Read the model definition and answer for the solid it produces. Units are mm, in the model's axes. Coordinates: 2 decimals unless noted, no trailing zeros. Write each loop counter-clockwise with the first axis right and the second up, starting at its lowest first coordinate (ties: lowest second). Pieces come first, ordered by that corner, then holes.
Item 1: Section A-A (x = 177) is taken. Give the vertices of the cut face in (y, z).
Item 2: Straight lines are drawn through the part: probe 1 along X at (y, z) = (35, 52.5); probe 2 along Y at (x, z) = (214.5, 45); probe 3 along Z at (x, y) = (-800.1, 36.1). For each, find the intervals that lie inside material, in ascending order.
Item 3: Each of these flat-tipped pins is pushed along its axis until it touches: P1, Ø4.5, axis at x = 520.7, z = 52.98, coming from the -Y side; P2, Ø6, axis at x = -85.5, y = -12, coming from the +Z side. Where does it stop, or does it pass through?
Item 4: Section B-B (y = 6) is taken. Give the vertices of the cut face in (x, z).
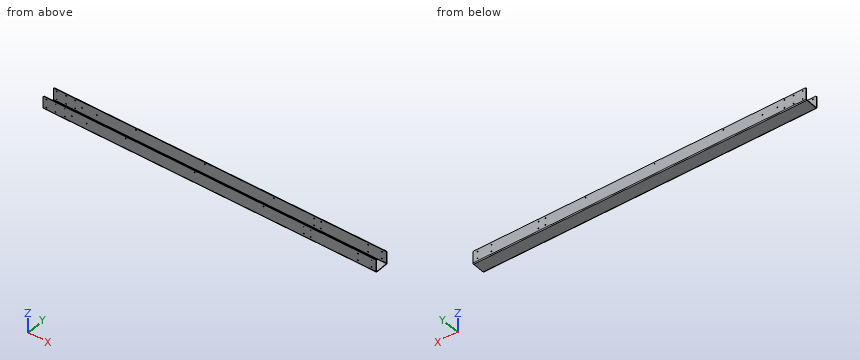
from build123d import *

# Parameters (mm, degrees)
SKETCH2_W                      = 1841.5
SKETCH2_H                      = 69.6722
BASE_FLANGE1_DEPTH             = 3.2639
EDGE_FLANGE1_STRIP_W           = 15.5956
EDGE_FLANGE1_STRIP_H           = 3.2639
EDGE_FLANGE1_STRIP_CUT_DEPTH   = 1841.5
EDGE_FLANGE1_STRIP_2_W         = 15.5956
EDGE_FLANGE1_STRIP_2_H         = 3.2639
EDGE_FLANGE1_STRIP_CUT_2_DEPTH = 1841.5
EDGE_FLANGE1_DEPTH             = 1841.5
EDGE_FLANGE1_BEND_DEPTH        = 1841.5
F_10_0_1935_DIAMETER_HOLE1_D   = 4.9149
F_10_0_1935_DIAMETER_HOLE3_D   = 4.9149
F_10_0_1935_DIAMETER_HOLE4_D   = 4.9149
F_10_0_2_DIAMETER_HOLE1_D      = 5.08
F_10_0_1935_DIAMETER_HOLE6_D   = 4.9149
LPATTERN2_COUNT                = 3
LPATTERN2_PITCH                = 381
FILLET2_R                      = 6.35


# Sheet-metal steps are written as plain solids
with BuildPart() as part:
    # Sketch2 → Base-Flange1 (new body)
    with BuildSketch(Plane.XY):
        Rectangle(SKETCH2_W, SKETCH2_H)
    extrude(amount=-BASE_FLANGE1_DEPTH)

    # Edge-Flange1 strip (across the edge) → Edge-Flange1 strip cut (cut)
    with BuildSketch(Plane(origin=(920.75, 34.8361, 0), x_dir=(0, -1, 0), z_dir=(-1, 0, 0))):
        with Locations((-6.5278, -1.63195)):
            Rectangle(EDGE_FLANGE1_STRIP_W, EDGE_FLANGE1_STRIP_H)
    extrude(amount=EDGE_FLANGE1_STRIP_CUT_DEPTH, mode=Mode.SUBTRACT)

    # Edge-Flange1 strip 2 (across the edge) → Edge-Flange1 strip cut 2 (cut)
    with BuildSketch(Plane(origin=(-920.75, -34.8361, 0), x_dir=(0, 1, 0), z_dir=(1, 0, 0))):
        with Locations((-6.5278, -1.63195)):
            Rectangle(EDGE_FLANGE1_STRIP_2_W, EDGE_FLANGE1_STRIP_2_H)
    extrude(amount=EDGE_FLANGE1_STRIP_CUT_2_DEPTH, mode=Mode.SUBTRACT)

    # Edge-Flange1 section (across the edge) → Edge-Flange1 (add)
    with BuildSketch(Plane(origin=(920.75, 34.8361, 0), x_dir=(0, -1, 0), z_dir=(-1, 0, 0))):
        with BuildLine():
            Line((-3.2639, 1.27), (-3.2639, 66.5861))
            Line((-3.2639, 66.5861), (0, 66.5861))
            Line((0, 66.5861), (0, 1.27))
            ThreePointArc((0, 1.27), (0.371974388, 0.371974388), (1.27, 0))
            Line((1.27, 0), (1.27, -3.2639))
            ThreePointArc((1.27, -3.2639), (-1.935951435, -1.935951435), (-3.2639, 1.27))
        make_face()
    extrude(amount=EDGE_FLANGE1_DEPTH)

    # Edge-Flange1 section 2 (across the edge) → Edge-Flange1 bend (add)
    with BuildSketch(Plane(origin=(-920.75, -34.8361, 0), x_dir=(0, 1, 0), z_dir=(1, 0, 0))):
        with BuildLine():
            Line((-3.2639, 1.27), (-3.2639, 66.5861))
            Line((-3.2639, 66.5861), (0, 66.5861))
            Line((0, 66.5861), (0, 1.27))
            ThreePointArc((0, 1.27), (0.371974388, 0.371974388), (1.27, 0))
            Line((1.27, 0), (1.27, -3.2639))
            ThreePointArc((1.27, -3.2639), (-1.935951435, -1.935951435), (-3.2639, 1.27))
        make_face()
    extrude(amount=EDGE_FLANGE1_BEND_DEPTH)

    # #10 (0.1935) Diameter Hole1 (through all)
    with Locations(Plane(origin=(0, 38.1, 34.8361), x_dir=(-1, 0, 0), z_dir=(0, 1, 0))):
        with Locations((800.1, -23.13305), (800.1, 21.31695), (850.9, 21.31695), (850.9, -23.13305), (901.7, 21.31695), (901.7, -23.13305)):
            Hole(F_10_0_1935_DIAMETER_HOLE1_D / 2)

    # #10 (0.1935) Diameter Hole3 (through all)
    with Locations(Plane(origin=(0, 38.1, 0), x_dir=(1, 0, 0), z_dir=(0, 1, 0))):
        with Locations((819.15, -14.87805), (819.15, -52.97805), (895.35, -14.87805), (895.35, -52.97805)):
            Hole(F_10_0_1935_DIAMETER_HOLE3_D / 2)

    # #10 (0.1935) Diameter Hole4 (through all)
    with Locations(Plane(origin=(0, 38.1, 0), x_dir=(1, 0, 0), z_dir=(0, 1, 0))):
        with Locations((520.7, -14.87805), (558.8, -14.87805), (558.8, -52.97805), (520.7, -52.97805)):
            Hole(F_10_0_1935_DIAMETER_HOLE4_D / 2)

    # #10 (0.2) Diameter Hole1 (through all)
    with Locations(Plane(origin=(0, 38.1, 0), x_dir=(1, 0, 0), z_dir=(0, 1, 0))):
        with Locations((-761.32055, -33.92805), (-678.77055, -33.92805)):
            Hole(F_10_0_2_DIAMETER_HOLE1_D / 2)

    # #10 (0.1935) Diameter Hole6 (through all)
    with Locations(Plane(origin=(0, -38.1, 0), x_dir=(-1, 0, 0), z_dir=(0, -1, 0))):
        with Locations((463.55, -57.0611)):
            f_10_0_1935_diameter_hole6 = Hole(F_10_0_1935_DIAMETER_HOLE6_D / 2)

    # LPattern2: #10 (0.1935) Diameter Hole6 ×3
    with Locations(*[(i * LPATTERN2_PITCH, 0, 0) for i in range(1, LPATTERN2_COUNT)]):
        add(f_10_0_1935_diameter_hole6, mode=Mode.SUBTRACT)

    # Fillet2
    fillet2_edges = [part.edges().sort_by_distance(p)[0] for p in [
        (920.75, 36.46805, 66.5861),
        (-920.75, 36.46805, 66.5861),
        (-920.75, -36.46805, 66.5861),
        (920.75, -36.46805, 66.5861),
    ]]
    fillet(fillet2_edges, radius=FILLET2_R)


solid = part.part
Established:
1. outline: (-38.1, 1.27) arc R4.53 ccw to (-33.57, -3.26) - (33.57, -3.26) arc R4.53 ccw to (38.1, 1.27) - (38.1, 66.59) - (34.84, 66.59) - (34.84, 1.27) arc R1.27 cw to (33.57, 0) - (-33.57, 0) arc R1.27 cw to (-34.84, 1.27) - (-34.84, 66.59) - (-38.1, 66.59) - close
2. probe 1: x = -920.75 to 518.29, 523.11 to 556.39, 561.21 to 816.74, 821.56 to 892.94, 897.76 to 920.75
2. probe 2: y = -38.1 to -34.84, 34.84 to 38.1
2. probe 3: z = -2.49 to 9.25, 14.16 to 53.7, 58.61 to 66.59
3. P1: passes through
3. P2: stops at z = 0
4. outline: (-920.75, -3.26) - (920.75, -3.26) - (920.75, 0) - (-920.75, 0) - close
